```python
from build123d import *

# Parameters (mm, degrees)
SKETCH1_W           = 17.78
SKETCH1_H           = 30.734
BOSS_EXTRUDE1_DEPTH = 2.54
SKETCH2_W           = 17.78
SKETCH2_H           = 5.08
BOSS_EXTRUDE2_DEPTH = 5.08
SKETCH3_W           = 17.78
SKETCH3_H           = 2.54
BOSS_EXTRUDE3_DEPTH = 5.08
SKETCH4_W           = 17.78
SKETCH4_H           = 9.8044
BOSS_EXTRUDE4_DEPTH = 4.826
SKETCH5_W           = 17.78
SKETCH5_H           = 2.286
BOSS_EXTRUDE5_DEPTH = 4.826


with BuildPart() as part:
    # Sketch1 → Boss-Extrude1 (new body)
    with BuildSketch(Plane.XY):
        Rectangle(SKETCH1_W, SKETCH1_H)
    extrude(amount=BOSS_EXTRUDE1_DEPTH)

    # Sketch2 → Boss-Extrude2 (add)
    with BuildSketch(Plane.XY.offset(2.54)):
        with Locations((0, -12.827)):
            Rectangle(SKETCH2_W, SKETCH2_H)
    boss_extrude2 = extrude(amount=BOSS_EXTRUDE2_DEPTH)

    # Sketch3 → Boss-Extrude3 (add)
    with BuildSketch(Plane(origin=(0, -10.287, 0), x_dir=(1, 0, 0), z_dir=(0, 1, 0))):
        with Locations((0, -6.35)):
            Rectangle(SKETCH3_W, SKETCH3_H)
    boss_extrude3 = extrude(amount=BOSS_EXTRUDE3_DEPTH)

    # Mirror1: Boss-Extrude2, Boss-Extrude3 across plane
    add(boss_extrude2.mirror(Plane.ZX))
    add(boss_extrude3.mirror(Plane.ZX))

    # Sketch4 → Boss-Extrude4 (add)
    with BuildSketch(Plane(origin=(0, 0, 0), x_dir=(-1, 0, 0), z_dir=(0, 0, -1))):
        Rectangle(SKETCH4_W, SKETCH4_H)
    boss_extrude4 = extrude(amount=BOSS_EXTRUDE4_DEPTH)

    # Sketch5 → Boss-Extrude5 (add)
    with BuildSketch(Plane(origin=(0, 4.9022, 0), x_dir=(1, 0, 0), z_dir=(0, 1, 0))):
        with Locations((0, 3.683)):
            Rectangle(SKETCH5_W, SKETCH5_H)
    boss_extrude5 = extrude(amount=BOSS_EXTRUDE5_DEPTH)

    # Mirror2: Boss-Extrude4, Boss-Extrude5 across plane
    add(boss_extrude4.mirror(Plane.ZX))
    add(boss_extrude5.mirror(Plane.ZX))


solid = part.part
```
Build history of the part. All positions in model axes, mm. A direction names the side the tool comes from. Give positions to 0.01 mm unless a question says otherwise; leave off trailing zeros. Order: outer loops, then holes, each group sorted by start corner. A loop starts at its lowest first (then second) coordinate and runs counter-clockwise, first axis right, second up. Notation, with made-up numbers: M 43,41.5 L 72,41.5 A30 cw 72,74.5 Z; hole C 64,21 d2. An arc over 180 degrees is marked long. Write item = value, one per line. Start each with the question number.
(1) Slice it at D-D on z = 6. Write the cut outline in (x, y), plus the area to 3 significant figures.
(2) Pin check, flat tips, straight feed: pin 1 Ø1.5 at (x, y) = (-3.5, 0) entering from +Z; pin 2 Ø6 at (x, y) = (-0.5, 3.5) entering from +Z; pin 3 Ø0.7 at (x, z) = (-0.5, -3.5) entering from -Y; pin 4 Ø1.8 at (x, z) = (-2, -4) entering from +Y. Stop position of each tip, or through.
(3) Which spindle directions (+Z, -Z, +X, -X, +Y, -Y) get a long thin tool onto all of the face, cutting with end or side? Do faces 5 (the flat face through (0, 10.287, 4)), 6 (the flat face through (0, 9.728, -4)), 7 (the flat face through (0, -4.902, -1)), 8 (the flat face through (0, 10, 0)). Say none if no direction does.
(4) Slice it at B-B on y = 6.5. Write the cut outline in (x, z), plus the area to 3 significant figures.
(5) Slice it at C-C on x = -6. Write the cut outline in (y, z), plus the area to 3 significant figures.
(6) Two-plate mould, pull along Y, no slides. Class faces 1 (the flat face through (0, -15.367, 4)), 2 (the flat face through (0, 5.207, 6)), 3 (the flat face through (0, 15.367, 4)), 4 (the flat face through (0, 0, -4.826)): released by +Y, released by -Y, zero draft, split by the parting line, or undercut.
(7) Probe L1, parallel to Z at x = -2.75, y = 7.5; L2, parallel to Z at x = 5, y = 10; L3, parallel to Y at x = -3, z = 5. List the from-to ranges inside material, lowest first. Write a range as [from, to].
(8) Slice it at A-A on z = 4.5. Write the cut outline in (x, y).
Responses:
q1.outline = M -8.89,-15.37 L 8.89,-15.37 L 8.89,-5.21 L -8.89,-5.21 Z; M -8.89,5.21 L 8.89,5.21 L 8.89,15.37 L -8.89,15.37 Z
q1.area = 361 mm2
q2.pin_1 = 2.54
q2.pin_2 = 7.62
q2.pin_3 = -9.73
q2.pin_4 = 9.73
q3.face_5 = +X, -X
q3.face_6 = -Z, +X, -X, +Y
q3.face_7 = +X, -X, -Y
q3.face_8 = +X, -X, +Y
q4.outline = M -8.89,-4.83 L 8.89,-4.83 L 8.89,-2.54 L -8.89,-2.54 Z; M -8.89,0 L 8.89,0 L 8.89,2.54 L -8.89,2.54 Z; M -8.89,5.08 L 8.89,5.08 L 8.89,7.62 L -8.89,7.62 Z
q4.area = 131 mm2
q5.outline = M -15.37,0 L -4.9,0 L -4.9,-2.54 L -9.73,-2.54 L -9.73,-4.83 L 9.73,-4.83 L 9.73,-2.54 L 4.9,-2.54 L 4.9,0 L 15.37,0 L 15.37,7.62 L 5.21,7.62 L 5.21,5.08 L 10.29,5.08 L 10.29,2.54 L -10.29,2.54 L -10.29,5.08 L -5.21,5.08 L -5.21,7.62 L -15.37,7.62 Z
q5.area = 225 mm2
q6.face_1 = released by -Y
q6.face_2 = undercut
q6.face_3 = released by +Y
q6.face_4 = zero draft
q7.L1 = [-4.83, -2.54], [0, 2.54], [5.08, 7.62]
q7.L2 = [0, 2.54], [5.08, 7.62]
q7.L3 = [-15.37, -10.29], [10.29, 15.37]
q8.outline = M -8.89,-15.37 L 8.89,-15.37 L 8.89,-10.29 L -8.89,-10.29 Z; M -8.89,10.29 L 8.89,10.29 L 8.89,15.37 L -8.89,15.37 Z
